Input: dimensioned drawing with shaded views. Units: mm. Origin: part minimum x, y, z. A direction names the side the tool comes from. Round coordinates to 2 decimals unless told otherwise and drop trailing zeros. Loops run counter-clockwise (first coordinate to the right, second up) from the corner with the lowest first, then second, coordinate; pieces in that order, holes last.
Item 1: First-contact query: P1, Ø7, axis at x = 13, y = 13, coming from the +Z side; P2, Ø1, axis at y = 22, z = 5, coming from the +X side. Flat tips, straight axial feed; report the tip coordinate or a pass-through.
Item 2: Section query D-D on y = 9.75. Return loops of the section in (x, z).
Item 3: Access query for the marked faces 1 and 2. Directions: +Z, -Z, +X, -X, +Y, -Y. A direction counts if a zero-diameter tool reaches every point of the face in a straight line with its end or side. Return the directions, or none.
Item 4: Section query A-A on y = 13. Return loops of the section in (x, z), then the cut area to 3 significant figures.
Item 5: Section query C-C on z = 8. Return loops of the section in (x, y), then the cut area to 3 significant figures.
Item 6: Ray query, L1, parallel to Y at x = 13, z = 3.1; L2, parallel to Y at x = 13, z = 8.5; L3, parallel to Z at x = 16.5, y = 11. Return the intervals inside material, ascending.
Item 7: Pull-direction query (X, two-part tool) for the marked faces 3, 4, 5 and 6; classes: released by +X, released by -X, zero draft, split by the parting line, or undercut.
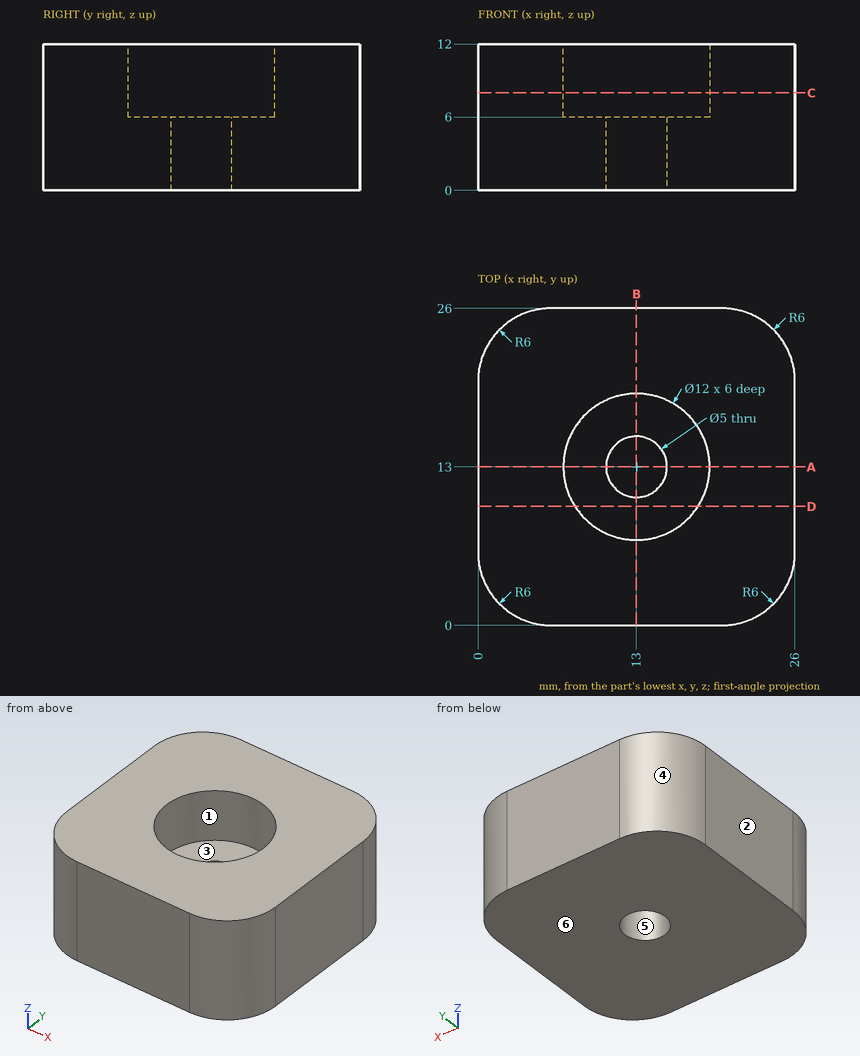
Data:
1. P1: stops at z = 6
1. P2: stops at x = 25.81
2. outline: (0, 0) - (26, 0) - (26, 12) - (18.04, 12) - (18.04, 6) - (7.96, 6) - (7.96, 12) - (0, 12) - close
3. face 1: +Z
3. face 2: +Z, -Z, -X, +Y, -Y
4. outline: (0, 0) - (10.5, 0) - (10.5, 6) - (7, 6) - (7, 12) - (0, 12) - close; (15.5, 0) - (26, 0) - (26, 12) - (19, 12) - (19, 6) - (15.5, 6) - close
4. area: 210 mm2
5. outline: (0, 6) arc R6 ccw to (6, 0) - (20, 0) arc R6 ccw to (26, 6) - (26, 20) arc R6 ccw to (20, 26) - (6, 26) arc R6 ccw to (0, 20) - close; hole circle Ø12 at (13, 13)
5. area: 532 mm2
6. L1: y = 0 to 10.5, 15.5 to 26
6. L2: y = 0 to 7, 19 to 26
6. L3: z = 0 to 6
7. face 3: undercut
7. face 4: released by -X
7. face 5: undercut
7. face 6: zero draft
